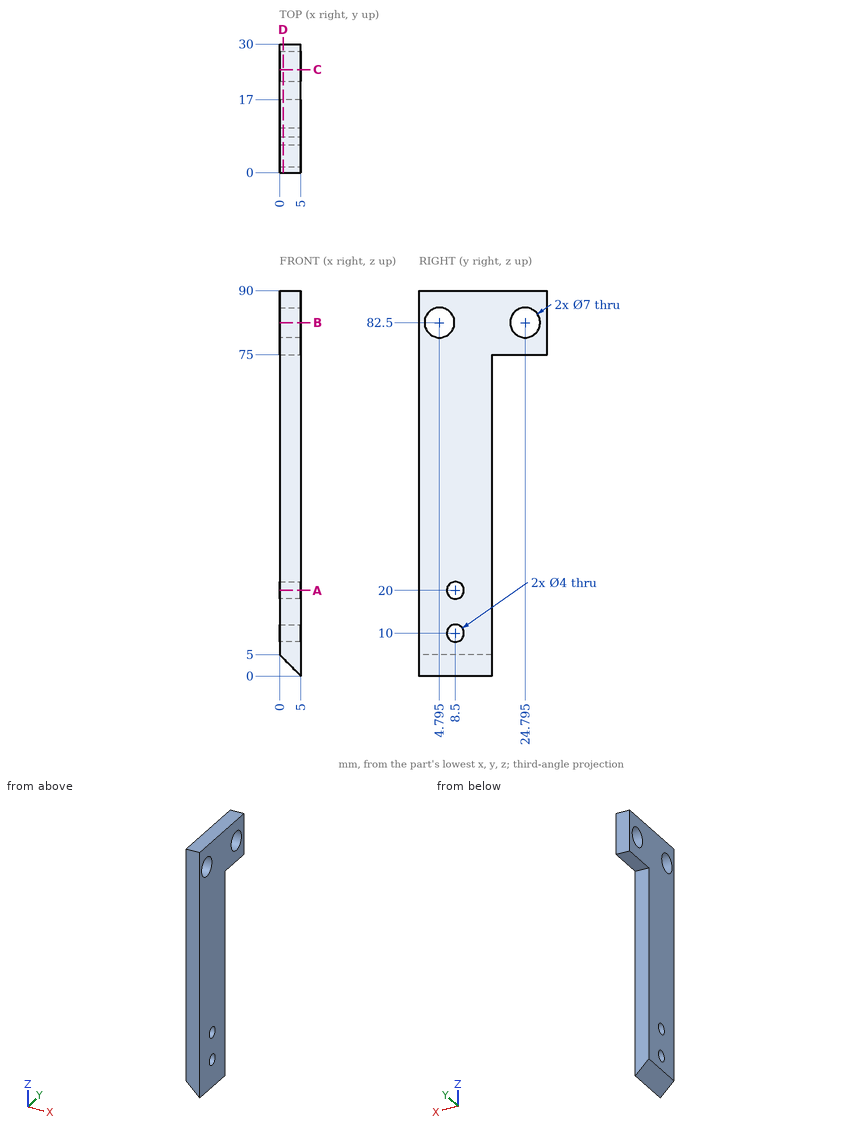
Verification items for this drawing (mm, ordinates from the low corner). Coordinates: 2 decimals unless noted, no trailing zeros. Order: outer loops, then holes, each group sorted by start corner. A loop starts at its lowest first (then second) coordinate and runs counter-clockwise, first axis right, second up. Notation, with made-up numbers: (44, 31.5) -> (75, 31.5) arc R9 ccw to (75, 48.5) -> close; hole circle Ø2 at (39, -18.75). An arc over 180 degrees is marked (long way). Put each result on its own line as item: value. Start each with the question number.
1. Cross-section at D-D, the plane x = 0.85. Record the boundary of the cut face in (y, z) (3 decimals), then the cut area to 3 significant figures.
2. Cross-section at C-C, the plane y = 24. Record the boundary of the cut face in (x, z).
3. Go/stop test with flat-tipped pins: pin 1 Ø6.5 at (y, z) = (4.8, 82.5) entering from -X; pin 2 Ø2.5 at (x, y) = (2, 25.5) entering from -Z; pin 3 Ø1.5 at (y, z) = (19, 79.5) entering from -X. Record where each tip stops, or that it passes through.
4. Material ranges on L1, parallel to Y at x = 1.95, z = 82.5 (3 decimals); L2, parallel to Z at x = 4.75, y = 2; L3, parallel to Y at x = 2.1, z = 26, recorded low to high. Write a range as [from, to].
5. Cross-section at B-B, the plane z = 82.5. Record the boundary of the cut face in (x, y) (3 decimals), then the cut area to 3 significant figures.
6. Cross-section at A-A, the plane z = 20. Record the boundary of the cut face in (x, y).
Computed:
1. outline: (0, 4.15) -> (17, 4.15) -> (17, 75) -> (30, 75) -> (30, 90) -> (0, 90) -> close; hole circle Ø7 at (4.795, 82.5); hole circle Ø4 at (8.5, 10); hole circle Ø4 at (8.5, 20); hole circle Ø7 at (24.795, 82.5)
1. area: 1,550 mm2
2. outline: (0, 75) -> (5, 75) -> (5, 79.09) -> (0, 79.09) -> close; (0, 85.91) -> (5, 85.91) -> (5, 90) -> (0, 90) -> close
3. pin 1: through
3. pin 2: z = 75
3. pin 3: x = 0
4. L1: [0, 1.295], [8.295, 21.295], [28.295, 30]
4. L2: [0.25, 80.39], [84.61, 90]
4. L3: [0, 17]
5. outline: (0, 0) -> (5, 0) -> (5, 1.295) -> (0, 1.295) -> close; (0, 8.295) -> (5, 8.295) -> (5, 21.295) -> (0, 21.295) -> close; (0, 28.295) -> (5, 28.295) -> (5, 30) -> (0, 30) -> close
5. area: 80.0 mm2
6. outline: (0, 0) -> (5, 0) -> (5, 6.5) -> (0, 6.5) -> close; (0, 10.5) -> (5, 10.5) -> (5, 17) -> (0, 17) -> close
